Can you work these out from the model? Positions are in its coordinate system, mm. Face numbers are marked on the shaded views. A direction names the side the tool comes from. Give positions to 0.01 mm unless a question says otherwise; leave off trailing zeros. Write each loop counter-clockwise with the first axis right and the second up, starting at its lowest first coordinate (ties: lowest second). Pieces come first, ordered by that corner, then holes. Notation, with made-up numbers: M -11,-0.75 L 0,-0.75 A25 ccw 0,11.25 Z; hole C 0,-20 d6. An arc over 180 degrees is marked long. Write each question's results on one line, items separated by ' | '.
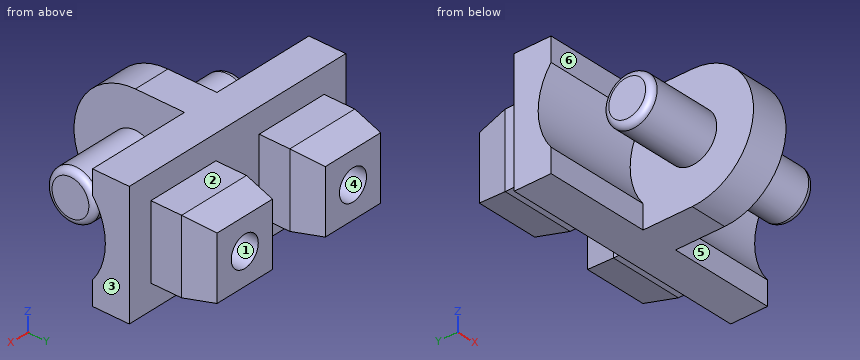
from build123d import *

# Parameters (mm, degrees)
LEG_CONNECTOR_DEPTH                            = 1.5
TORSO_CONNECTOR_DEPTH                          = 8.5
SKETCH3_R                                      = 2
LEG_PIN_DEPTH                                  = 6
SKETCH4_W                                      = 6
SKETCH4_H                                      = 6
TORSO_PIN_BASE_DEPTH                           = 2.5
SKETCH5_W                                      = 6
SKETCH5_H                                      = 6
TORSO_PIN_TIP_DEPTH                            = 2.5
TORSO_PIN_TIP_TAPER                            = 10
HOLE_THAT_MAKE_IT_EASY_TO_ADD_CENTER_LIN_D     = 2.5
HOLE_THAT_MAKE_IT_EASY_TO_ADD_CENTER_LIN_DEPTH = 3.5
HOLE_THAT_MAKE_IT_EASY_TO_ADD_CENTER_LIN_TIP   = 0.751075774
EASY_LEG_INSERT_R                              = 0.5
SCALE1_SCALE                                   = 2


with BuildPart() as part:
    # Sketch1 → Leg connector (new body)
    with BuildSketch(Plane(origin=(0, 0, 0), x_dir=(0, 0, -1), z_dir=(1, 0, 0))):
        with BuildLine():
            Line((-5, 0), (5, 0))
            Line((5, 0), (5, -7))
            ThreePointArc((5, -7), (0, -12), (-5, -7))
            Line((-5, -7), (-5, 0))
        make_face()
    extrude(amount=LEG_CONNECTOR_DEPTH)

    # Sketch2 → Torso connector (add)
    with BuildSketch(Plane(origin=(1.5, 0, 0), x_dir=(0, 0, -1), z_dir=(1, 0, 0))):
        with BuildLine():
            Line((-5, 0), (5, 0))
            Line((5, 0), (5, -3))
            Line((5, -3), (3.082612528, -3))
            ThreePointArc((3.082612528, -3), (0, -1.95), (-3.082612528, -3))
            Line((-3.082612528, -3), (-5, -3))
            Line((-5, -3), (-5, 0))
        make_face()
    extrude(amount=TORSO_CONNECTOR_DEPTH)

    # Sketch3 → Leg pin (add)
    with BuildSketch(Plane(origin=(1.5, 0, 0), x_dir=(0, 0, -1), z_dir=(1, 0, 0))):
        with Locations((0, -7)):
            Circle(SKETCH3_R)
    extrude(amount=LEG_PIN_DEPTH)

    # Sketch4 → Torso pin base (add)
    with BuildSketch(Plane(origin=(0, 0, 0), x_dir=(1, 0, 0), z_dir=(0, 1, 0))):
        with Locations((5, 0)):
            Rectangle(SKETCH4_W, SKETCH4_H)
    extrude(amount=TORSO_PIN_BASE_DEPTH)

    # Sketch5 → Torso pin tip (add)
    with BuildSketch(Plane(origin=(0, 2.5, 0), x_dir=(1, 0, 0), z_dir=(0, 1, 0))):
        with Locations((5, 0)):
            Rectangle(SKETCH5_W, SKETCH5_H)
    extrude(amount=TORSO_PIN_TIP_DEPTH, taper=TORSO_PIN_TIP_TAPER)

    # Hole that make it easy to add center lines
    with Locations(Plane(origin=(0, 5, 0), x_dir=(1, 0, 0), z_dir=(0, 1, 0))):
        with Locations((5, 0)):
            Hole(HOLE_THAT_MAKE_IT_EASY_TO_ADD_CENTER_LIN_D / 2, depth=HOLE_THAT_MAKE_IT_EASY_TO_ADD_CENTER_LIN_DEPTH)
            with Locations((0, 0, -(HOLE_THAT_MAKE_IT_EASY_TO_ADD_CENTER_LIN_DEPTH + HOLE_THAT_MAKE_IT_EASY_TO_ADD_CENTER_LIN_TIP / 2))):  # 118° drill point
                Cone(0, HOLE_THAT_MAKE_IT_EASY_TO_ADD_CENTER_LIN_D / 2, HOLE_THAT_MAKE_IT_EASY_TO_ADD_CENTER_LIN_TIP, mode=Mode.SUBTRACT)

    # Easy leg insert
    easy_leg_insert_edges = [part.edges().sort_by_distance(p)[0] for p in [
        (7.5, -7, 2),
    ]]
    fillet(easy_leg_insert_edges, radius=EASY_LEG_INSERT_R)

    # Making symetrical: part across plane


with BuildPart() as part_1:
    add(part.part)
    add(part.part.mirror(Plane(origin=(0, -7, 0), x_dir=(0, 0, 1), z_dir=(1, 0, 0))))


with BuildPart() as part_2:
    # Scale1: scaled about (0, -2.270029125, 0)
    add(part_1.part.scale(SCALE1_SCALE).moved(Location((0, 2.270029125, 0))))


solid = part_2.part
Item 1: For the marked faces 4, 5 and 6, which set-ups out of +Z, -Z, +X, -X, +Y, -Y let a thin tool reach every point of the face, with its end or its side?
Geometry says:
face 4: +Y | face 5: +Z, -Z, +X, -Y | face 6: +Z, -Z, -X, -Y
Item 2: If I drill on line 1 (X direction, y = 6, z = -1.75); line 2 (Z direction, x = -10, y = 7); line 3 (X direction, y = 11, z = -0.5), over which ranges is the centre line in solid material (lowest first)? Write a range as from..to.
Geometry says:
line 1: x = -16..-11.79, -8.21..-4, 4..8.21, 11.79..16 | line 2: z = -6..-2.5, 2.5..6 | line 3: x = -15.34..-12.45, -7.55..-4.66, 4.66..7.55, 12.45..15.34
Item 3: I'm going to push flat-ended pins straight in: pin 1 (1.5 mm diameter, centred on y = 4.5, z = 2.5, fed in from -X); pin 2 (4 mm diameter, centred on x = -10, z = 0, fed in from +Y); pin 3 (1 mm diameter, centred on y = -6.5, z = 2, fed in from -X). Where does each tip first touch, or does it pass through?
Geometry says:
pin 1: stops at x = -16 | pin 2: stops at y = 4.97 | pin 3: stops at x = -3
Item 4: Thinking about a two-plate mould opening in X: for the marked faces 1, 2 and 3, which applies, +X half, -X half, draft (parallel to the pull), parting line (faces both ways), or undercut?
Geometry says:
face 1: undercut | face 2: draft | face 3: +X half
Item 5: I want a section at A-A, the plane z = -8. Please give me the cut outline in (x, y), and give its area (3 significant figures).
Geometry says:
outline: M -20,-3.73 L -3,-3.73 L -3,-17.73 L 3,-17.73 L 3,-3.73 L 20,-3.73 L 20,2.27 L -20,2.27 Z | area: 324 mm2
Item 6: I want a section at B-B, the plane y = -7. Please give me the cut outline in (x, z), and give its area (3 significant figures).
Geometry says:
outline: M -3,-10 L 3,-10 L 3,10 L -3,10 Z | area: 120 mm2
Item 7: I want a section at D-D, the plane z = 8.75. Please give me the cut outline in (x, y), and give its area (3 significant figures).
Geometry says:
outline: M -20,-3.73 L -3,-3.73 L -3,-16.57 L 3,-16.57 L 3,-3.73 L 20,-3.73 L 20,2.27 L -20,2.27 Z | area: 317 mm2
Item 8: I want a section at C-C, the plane x = 1. Please give me the cut outline in (y, z).
Geometry says:
outline: M -11.73,-10 L 2.27,-10 L 2.27,10 L -11.73,10 A10 ccw Z
